from build123d import *

# Parameters (mm, degrees)
F0_W     = 101.6
F0_H     = 76.2
F1_DEPTH = 25.4
F3_DEPTH = 25.4
F5_DEPTH = 25.4


with BuildPart() as f1:
    # F0 (on Top) → F1 (new body)
    with BuildSketch(Plane.XY):
        with Locations((-2.444915, -13.285797)):
            Rectangle(F0_W, F0_H)
    extrude(amount=F1_DEPTH)

    # F2 (on face) → F3 (join)
    with BuildSketch(Plane.XY.offset(25.4)):
        Polygon((-53.244915, 24.814203), (-53.244915, -51.385797), (-40.544915, -51.385797), (10.255085, 24.814203), align=None)
    extrude(amount=F3_DEPTH)

    # F4 (on face) → F5 (join)
    with BuildSketch(Plane.XY.offset(25.4)):
        Polygon((22.955085, -51.385797), (48.355085, -51.385797), (48.355085, -13.285797), (39.337236, -13.285797), align=None)
    extrude(amount=F5_DEPTH)


solid = f1.part
Verification items for the finished model (mm, model axes). A direction names the side the tool comes from. Give positions to 0.01 mm unless a question says otherwise; leave off trailing zeros. Loops run counter-clockwise (first coordinate to the right, second up) from the corner with the lowest first, then second, coordinate; pieces in that order, holes last. Notation, with made-up numbers: (12.5, -18.5) - (19.5, -18.5) arc R13 ccw to (19.5, 6.5) - close; hole circle Ø4 at (-29, 53.5). An arc over 180 degrees is marked (long way). Write item = value, one per line. Start each with the question number.
Q1. Thickness scan on line 1 (Z direction, x = 16.5, y = -22); line 2 (X direction, y = -10.5, z = 31); line 3 (X direction, y = -36, z = 32). Record the ranges inside material, lowest first.
Q2. Cross-section at D-D, the plane x = -26. Enter the section's corners in (y, z).
Q3. Cross-section at B-B, the plane y = 8. Enter the section's corners in (x, z).
Q4. Cross-section at C-C, the plane x = 19.5. Enter the section's corners in (y, z), and give its area (3 significant figures).
Q5. Cross-section at A-A, the plane z = 42.5. Enter the section's corners in (x, y).
Q6. Tool access check on faces 1 (the face through (-15.5, -13.82, 37.92)), 2 (the face through (44, -13.286, 38)), 3 (the face through (31.26, -32.07, 37.92)). Record the directions out of +Z, -Z, +X, -X, +Y, -Y that give a thin tool (end or side, any length) a straight path to the whole face; none if there is none.
Q7. Depth check by flat-ended pin: P1, Ø2, axis at x = 16, y = 9.5, coming from the +Z side; P2, Ø2.5, axis at x = 42, z = 35, coming from the +Y side. Enter the tip coordinate at first touch or a pass-through.
Q8. Mould release check, pull along X, two halves, no side actions. Record for faces 4 (the face through (13, -13, 25.4)), 5 (the face through (38, -36, 50.8)), 6 (the face through (-53.245, -13, 25)): released by +X, released by -X, zero draft, split by the parting line, or undercut.
Answer key:
q1.line_1 = 0 to 25.4
q1.line_2 = -53.24 to -13.29
q1.line_3 = -53.24 to -30.29, 29.57 to 48.36
q2.outline = (-51.39, 0) - (24.81, 0) - (24.81, 50.8) - (-29.57, 50.8) - (-29.57, 25.4) - (-51.39, 25.4) - close
q3.outline = (-53.24, 0) - (48.36, 0) - (48.36, 25.4) - (-0.95, 25.4) - (-0.95, 50.8) - (-53.24, 50.8) - close
q4.outline = (-51.39, 0) - (24.81, 0) - (24.81, 25.4) - (-51.39, 25.4) - close
q4.area = 1,940 mm^2
q5.outline = (-53.24, -51.39) - (-40.54, -51.39) - (10.26, 24.81) - (-53.24, 24.81) - close; (22.96, -51.39) - (48.36, -51.39) - (48.36, -13.29) - (39.34, -13.29) - close
q6.face_1 = +Z, -Y
q6.face_2 = +Z, +X, +Y
q6.face_3 = +Z, +Y
q7.P1 = 25.4
q7.P2 = -13.29
q8.face_4 = undercut
q8.face_5 = zero draft
q8.face_6 = released by -X
